Design review of the part shown in the three views and the two pictorial views. Dimensions are in mm from the part's minimum x, y and z. A direction names the side the tool comes from. Give positions to 0.01 mm unless a question says otherwise; leave off trailing zeros. Return JSON: item names as keys, results as strings. Group by question number.
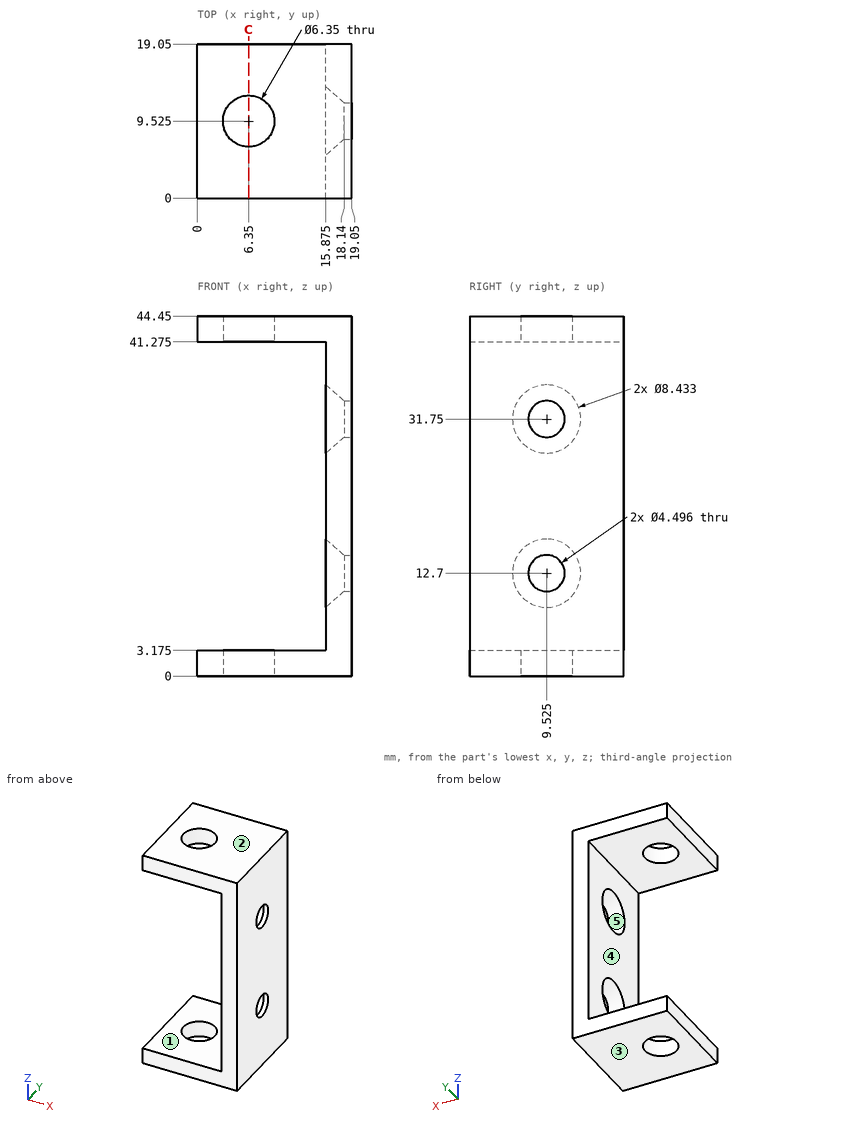
Item 1: For P1, Ø5.5, axis at x = 6.35, y = 9.525, coming from the +Z side; P2, Ø5.5, axis at y = 8, z = 17.5, coming from the -X side (1 decimal); P3, Ø7, axis at y = 9.525, z = 12.7, coming from the -X side; P4, Ø8, axis at y = 2.5, z = 37.5, coming from the -X side, all flat-tipped, find the tip position at first contact; note any pin that passes through.
Item 2: Take a section at C-C (x = 6.35). State how many separate pieces and enclosed holes the cut face has.
Item 3: Tool access review of the marked faces 4 and 5: name each direction out of +Z, -Z, +X, -X, +Y, -Y from which nothing blocks a thin tool from reaching the whole face with its end or side.
Item 4: For L1, parallel to Y at x = 18.55, z = 12.7; L2, parallel to X at y = 6.75, z = 32, list the stretches that pass through material, from the lowest coordinate up. Write a range as from..to.
Item 5: Mouldability with a two-part tool opening along Z and no side actions: class the marked faces 1, 2 and 3 as +Z half, -Z half, draft (parallel to the pull), parting line (faces both ways), or undercut.
Check sheet entries:
{
 "1": {"P1": "passes through", "P2": "stops at x = 15.9", "P3": "stops at x = 16.7", "P4": "stops at x = 0"},
 "2": {"separate pieces": "4", "enclosed holes": "0"},
 "3": {"face 4": "-X, +Y, -Y", "face 5": "-X"},
 "4": {"L1": "y = 0..7.28, 11.77..19.05", "L2": "x = 17.52..19.05"},
 "5": {"face 1": "undercut", "face 2": "+Z half", "face 3": "-Z half"}
}
